Autodesk Inventor part; units mm, degrees
ref_plane "YZ Plane" through (0, 0, 0) normal (1, 0, 0) x (0, 1, 0)
ref_plane "XZ Plane" through (0, 0, 0) normal (0, 1, 0) x (-1, 0, 0)
ref_plane "XY Plane" through (0, 0, 0) normal (0, 0, 1) x (1, 0, 0)
sketch "Sketch1" plane through (0, 0, 0) normal (0, 1, 0) x (-1, 0, 0)
  line L0 (0, 0) -> (0, -27.002) construction
  line L1 (19.064, 12.0028) -> (-19.064, 12.0028)
  line L2 (-19.064, 12.0028) -> (-19.064, -23.4972)
  line L3 (-19.064, -23.4972) -> (19.064, -23.4972)
  line L4 (19.064, -23.4972) -> (19.064, 12.0028)
  dimension "d0" = 35.5
  dimension "d12" = 38.128
extrude "Plate1" add sketch "Sketch1" along normal blind 5
sketch "Sketch2" plane through (-14.0762, 0.3488, 12.0028) normal (-0.9975641, -0.0697565, 0) x (0.0697565, -0.9975641, 0)
  line L0 (0, -35.5) -> (0, 0)
  line L1 (0, 0) -> (-21.37, 0)
  line L2 (-21.37, 0) -> (-21.37, -35.5)
  line L3 (-21.37, -35.5) -> (0, -35.5)
edge flange "Flange1" height 21.37 angle 86 thickness 5 bend radius 1 thickness toward (-0.9975641, -0.0697565, 0) relief tear relief width 5 relief depth 2.5 corner gap 1 corner form 0 edges at (-19.064, 5, -5.7472) (19.064, 5, -5.7472) wall of the first edge with corners at (-14.0762, 0.3488, -23.4972) (-14.0762, 0.3488, 12.0028) (-15.5669, 21.6667, 12.0028) (-15.5669, 21.6667, -23.4972)
bend "Bend1"
corner "Corner1"
equation "\"d1\" = Thickness"
equation "\"d2\" = BendReliefWidth"
equation "\"d3\" = BendReliefDepth"
equation "\"d4\" = MinimumRemnant"
equation "\"d5\" = TransitionRadius"
equation "\"d8\" = BendRadius"
equation "\"d9\" = CornerReliefSize"
equation "\"d10\" = GapSize"
equation "\"d11\" = JacobiRadiusSize"
equation "\"BendReliefWidth\" = Thickness"
equation "\"BendReliefDepth\" = 0.5 * Thickness"
equation "\"TransitionRadius\" = BendRadius"
equation "\"JacobiRadiusSize\" = BendRadius"
equation "\"GapSize\" = Thickness"
properties part number "øre" material "Steel"
Geometry check sheet. Reference: the model listing, model coordinates, mm. A direction names the side the tool comes from. Round coordinates to 2 decimals unless told otherwise and drop trailing zeros. Order: outer loops, then holes, each group sorted by start corner. A loop starts at its lowest first (then second) coordinate and runs counter-clockwise, first axis right, second up. Notation, with made-up numbers: M 19,27 L 46,27 A21 ccw 46,45 Z; hole C -40,80 d11. An arc over 180 degrees is marked long. Answer in a Markdown table with one row per item. Add a question column.
Item 1: Material ranges on L1, parallel to Y at x = 2, z = -2; L2, parallel to X at y = 14, z = -12; L3, parallel to X at y = 12.5, z = -17.5, recorded low to high. Write a range as [from, to].
Item 2: Set-up check for faces 5 (the face through (0, 4, -23.497)), 6 (the face through (15.01, 13.69, -6)): record each of +Z, -Z, +X, -X, +Y, -Y from which the full face is reachable in a straight line by a thin tool's end or side.
Item 3: Draft check along X on faces 1 (the face through (0, 5, -5)), 2 (the face through (0, 0, -5)), 3 (the face through (-18.026, 21.495, -5.499)), 4 (the face through (-15.01, 13.69, -5.5)). Enter one of: released by +X, released by -X, zero draft, split by the parting line, or undercut.
Item 4: Sectioned sample at D-D, the plane y = 2.25. Enter the section's corners in (x, z), plus the area to 3 significant figures.
Item 5: Depth check by flat-ended pin: pin 1 Ø8 at (x, z) = (0, 0) entering from +Y; pin 2 Ø1 at (x, y) = (13.5, 7) entering from +Z. Enter the tip coordinate at first touch or a pass-through.
Item 6: Sectioned sample at B-B, the plane z = -11.5. Enter the section's corners in (x, y), plus the area to 3 significant figures.
Item 7: Sectioned sample at A-A, the plane y = 17.5. Enter the section's corners in (x, z), plus the area to 3 significant figures.
Item 8: Sectioned sample at C-C, the plane x = 5. Enter the section's corners in (y, z), plus the area to 4 significant figures.
Filled in:
| question | item | result |
|---|---|---|
| 1 | L1 | y = [0, 5] |
| 1 | L2 | x = [-20.04, -15.03], [15.03, 20.04] |
| 1 | L3 | x = [-19.94, -14.93], [14.93, 19.94] |
| 2 | face 5 | -Z, +X, -X, +Y, -Y |
| 2 | face 6 | +Z, -Z, +Y |
| 3 | face 1 | undercut |
| 3 | face 2 | zero draft |
| 3 | face 3 | released by -X |
| 3 | face 4 | undercut |
| 4 | outline | M -18.15,-23.5 L 18.15,-23.5 L 18.15,12 L -18.15,12 Z |
| 4 | area | 1,290 mm² |
| 5 | pin 1 | stops at y = 5 |
| 5 | pin 2 | passes through |
| 6 | outline | M -20.55,21.32 L -19.45,5.58 A6 ccw -13.47,0 L 13.47,0 A6 ccw 19.45,5.58 L 20.55,21.32 L 15.57,21.67 L 14.47,5.93 A1 cw 13.47,5 L -13.47,5 A1 cw -14.47,5.93 L -15.57,21.67 Z |
| 6 | area | 345 mm² |
| 7 | outline | M -20.29,-23.5 L -15.28,-23.5 L -15.28,12 L -20.29,12 Z; M 15.28,-23.5 L 20.29,-23.5 L 20.29,12 L 15.28,12 Z |
| 7 | area | 356 mm² |
| 8 | outline | M 0,-23.5 L 5,-23.5 L 5,12 L 0,12 Z |
| 8 | area | 177.5 mm² |
